Work out the finished part from the listing and answer in its coordinate system (mm). Face numbers are marked on the shaded views. A direction names the side the tool comes from. Give positions to 0.01 mm unless a question says otherwise; leave off trailing zeros. Write each loop counter-clockwise with the first axis right and the second up, starting at its lowest first coordinate (ties: lowest second). Pieces come first, ordered by that corner, then holes. Notation, with made-up numbers: (39, 51.25) - (66, 51.25) arc R10 cw to (66, 68.25) - close; hole circle Ø3 at (-40, 31). An arc over 180 degrees is marked (long way). Write item = value, one per line.
from build123d import *

# Parameters (mm, degrees)
SKETCH1_R            = 33
SKETCH1_R_2          = 17.5
SKETCH1_W            = 7
SKETCH1_H            = 7
BOSS_EXTRUDE1_DEPTH  = 11
CUT_EXTRUDE1_START   = -12
CUT_EXTRUDE1_DEPTH   = 13
MIRROR2_START        = -12
MIRROR2_COPY_1_DEPTH = 13


with BuildPart() as part:
    # Sketch1 → Boss-Extrude1 (new body)
    with BuildSketch(Plane.XY):
        Circle(SKETCH1_R)
        Circle(SKETCH1_R_2, mode=Mode.SUBTRACT)
        Polygon((17.302558883, 11.468911087), (20.802558883, 17.531088913), (26.86473671, 14.031088913), (23.36473671, 7.968911087), align=None, mode=Mode.SUBTRACT)
        with Locations((25.5, 0)):
            Rectangle(SKETCH1_W, SKETCH1_H, mode=Mode.SUBTRACT)
        Polygon((7.968911087, 23.36473671), (14.031088913, 26.86473671), (17.531088913, 20.802558883), (11.468911087, 17.302558883), align=None, mode=Mode.SUBTRACT)
        with Locations((0, 25.5)):
            Rectangle(SKETCH1_W, SKETCH1_H, mode=Mode.SUBTRACT)
        with Locations((-25.5, 0)):
            Rectangle(SKETCH1_W, SKETCH1_H, mode=Mode.SUBTRACT)
        Polygon((-23.36473671, 7.968911087), (-26.86473671, 14.031088913), (-20.802558883, 17.531088913), (-17.302558883, 11.468911087), align=None, mode=Mode.SUBTRACT)
        Polygon((-11.468911087, 17.302558883), (-17.531088913, 20.802558883), (-14.031088913, 26.86473671), (-7.968911087, 23.36473671), align=None, mode=Mode.SUBTRACT)
        Polygon((23.36473671, -7.968911087), (26.86473671, -14.031088913), (20.802558883, -17.531088913), (17.302558883, -11.468911087), align=None, mode=Mode.SUBTRACT)
        Polygon((11.468911087, -17.302558883), (17.531088913, -20.802558883), (14.031088913, -26.86473671), (7.968911087, -23.36473671), align=None, mode=Mode.SUBTRACT)
        with Locations((0, -25.5)):
            Rectangle(SKETCH1_W, SKETCH1_H, mode=Mode.SUBTRACT)
        Polygon((-7.968911087, -23.36473671), (-11.468911087, -17.302558883), (-17.531088913, -20.802558883), (-14.031088913, -26.86473671), align=None, mode=Mode.SUBTRACT)
        Polygon((-17.302558883, -11.468911087), (-23.36473671, -7.968911087), (-26.86473671, -14.031088913), (-20.802558883, -17.531088913), align=None, mode=Mode.SUBTRACT)
    extrude(amount=BOSS_EXTRUDE1_DEPTH)

    # Sketch2 → Cut-Extrude1 (cut)
    with BuildSketch(Plane.XY.offset(11).offset(CUT_EXTRUDE1_START)):
        with BuildLine():
            Line((-195.710732602, 14.035729655), (-27.032017462, 18.9280224))
            ThreePointArc((-27.032017462, 18.9280224), (-21.370045373, 21.370045373), (-18.9280224, 27.032017462))
            Line((-18.9280224, 27.032017462), (-14.035729655, 195.710732602))
            Line((-14.035729655, 195.710732602), (-252.683769537, 434.358772484))
            Line((-252.683769537, 434.358772484), (-434.358772484, 252.683769537))
            Line((-434.358772484, 252.683769537), (-195.710732602, 14.035729655))
        make_face()
    cut_extrude1 = extrude(amount=CUT_EXTRUDE1_DEPTH, mode=Mode.SUBTRACT)

    # Mirror1: Cut-Extrude1 across plane
    add(cut_extrude1.mirror(Plane(origin=(0, 0, 0), x_dir=(0, 0, 1), z_dir=(1, 0, 0))), mode=Mode.SUBTRACT)

    # Mirror2: Cut-Extrude1 across plane
    add(cut_extrude1.mirror(Plane.ZX), mode=Mode.SUBTRACT)

    # Mirror2 copy 1 sketch → Mirror2 copy 1 (cut)
    with BuildSketch(Plane(origin=(0, 0, 11), x_dir=(-1, 0, 0), z_dir=(0, 0, 1)).offset(MIRROR2_START)):
        with BuildLine():
            Line((-195.710732602, 14.035729655), (-27.032017462, 18.9280224))
            ThreePointArc((-27.032017462, 18.9280224), (-21.370045373, 21.370045373), (-18.9280224, 27.032017462))
            Line((-18.9280224, 27.032017462), (-14.035729655, 195.710732602))
            Line((-14.035729655, 195.710732602), (-252.683769537, 434.358772484))
            Line((-252.683769537, 434.358772484), (-434.358772484, 252.683769537))
            Line((-434.358772484, 252.683769537), (-195.710732602, 14.035729655))
        make_face()
    extrude(amount=MIRROR2_COPY_1_DEPTH, mode=Mode.SUBTRACT)


solid = part.part
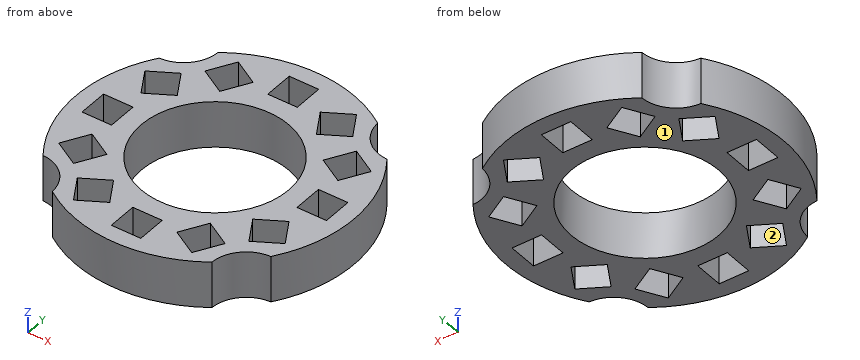
1. Find section C-C, the plane z = 6.5. Give the number of separate pieces and of enclosed holes in the cut face, then the cut area to 3 significant figures.
Solution:
separate_pieces = 1
enclosed_holes = 13
area = 1,780 mm^2
2. A tool of negligible diameter and unlimited length cuts with its end or side. For the marked faces 1 and 2, from which of +Z, -Z, +X, -X, +Y, -Y can it reach the whole face along a straight path? Write none if from no direction.
Solution:
face_1 = -Z, +X, -X, +Y, -Y
face_2 = +Z, -Z
3. Find section B-B, the plane y = -10.5. Give the vertices of the cut face in (x, z).
Solution:
outline = (-31.28, 0) - (-24.83, 0) - (-24.83, 11) - (-31.28, 11) - close; (-18.98, 0) - (-14, 0) - (-14, 11) - (-18.98, 11) - close; (14, 0) - (18.98, 0) - (18.98, 11) - (14, 11) - close; (24.83, 0) - (31.28, 0) - (31.28, 11) - (24.83, 11) - close
4. Given pin 1 (2 mm diameter, centred on y = -1.5, z = 6, fed in from +X); pin 2 (2 mm diameter, centred on x = 26.5, z = 4.5, fed in from -Y); pin 3 (10 mm diameter, centred on x = -5.5, y = -7.5, fed in from -Z); pin 4 (5.5 mm diameter, centred on x = -1, z = 4.5, fed in from -Y), each flat-ended and moving along its own axis, determine where each tip first touches the part or whether it passes through.
Solution:
pin_1 = 33
pin_2 = -19.12
pin_3 = through
pin_4 = -33
5. Straight lines are drawn through the part: line 1 (Y direction, x = 0, z = 8.25); line 2 (X direction, y = -16, z = 2.75); line 3 (X direction, y = 23, z = 6). For each, find the intervals that lie inside material, in ascending order.
Solution:
line_1 = -33 to -29, -22 to -17.5, 17.5 to 22, 29 to 33
line_2 = -28.86 to -23.45, -19.92 to -7.09, 7.09 to 19.92, 23.45 to 28.86
line_3 = -20.1 to -16.26, -8.18 to -3.5, 3.5 to 8.18, 16.26 to 20.1
6. Find section A-A, the plane x = 0. Give the vertices of the cut face in (y, z).
Solution:
outline = (-33, 0) - (-29, 0) - (-29, 11) - (-33, 11) - close; (-22, 0) - (-17.5, 0) - (-17.5, 11) - (-22, 11) - close; (17.5, 0) - (22, 0) - (22, 11) - (17.5, 11) - close; (29, 0) - (33, 0) - (33, 11) - (29, 11) - close
